```python
from build123d import *
from build123d.topology import SkipClean

# Parameters (mm, degrees)
SKETCH_1_R      = 1.9
SKETCH_1_R_2    = 2.7
SKETCH_1_R_3    = 2
EXTRUDE_1_DEPTH = 2.5
EXTRUDE_START   = -9
SKETCH_1_3_R    = 4.25
SKETCH_1_3_R_2  = 2.7
EXTRUDE_2_DEPTH = 9
SKETCH_2_R      = 3
SKETCH_2_R_2    = 1.9
EXTRUDE_4_DEPTH = 1
EXTRUDE_START_2 = 2.5
SKETCH_1_7_R    = 2.7
SKETCH_1_7_R_2  = 2
EXTRUDE_5_DEPTH = 10


with BuildPart() as part:
    # 草图1 → 凸台-拉伸1 (new body)
    with BuildSketch(Plane.XY):
        with BuildLine():
            ThreePointArc((-16.75, 33.05), (-19.75520382, 31.80520382), (-21, 28.8))
            Line((-21, 28.8), (-21, -28.8))
            ThreePointArc((-21, -28.8), (-19.75520382, -31.80520382), (-16.75, -33.05))
            Line((-16.75, -33.05), (16.75, -33.05))
            ThreePointArc((16.75, -33.05), (19.75520382, -31.80520382), (21, -28.8))
            Line((21, -28.8), (21, 28.8))
            ThreePointArc((21, 28.8), (19.75520382, 31.80520382), (16.75, 33.05))
            Line((16.75, 33.05), (-16.75, 33.05))
        make_face()
        with Locations((-12, 12)):
            Circle(SKETCH_1_R, mode=Mode.SUBTRACT)
        with Locations((-12, -12)):
            Circle(SKETCH_1_R, mode=Mode.SUBTRACT)
        with Locations((-16.75, 28.8)):
            Circle(SKETCH_1_R_2, mode=Mode.SUBTRACT)
        with Locations((-16.75, -28.8)):
            Circle(SKETCH_1_R_2, mode=Mode.SUBTRACT)
        with Locations((12, 12)):
            Circle(SKETCH_1_R, mode=Mode.SUBTRACT)
        with Locations((16.75, 28.8)):
            Circle(SKETCH_1_R_2, mode=Mode.SUBTRACT)
        with Locations((12, -12)):
            Circle(SKETCH_1_R, mode=Mode.SUBTRACT)
        with Locations((16.75, -28.8)):
            Circle(SKETCH_1_R_2, mode=Mode.SUBTRACT)
        Circle(SKETCH_1_R_3, mode=Mode.SUBTRACT)
    extrude(amount=EXTRUDE_1_DEPTH)

    # 草图1<3> → 凸台-拉伸2 (add)
    # profile 1 of 4: a face of its own
    with SkipClean():  # the faces are left unmerged after this step: merging them gives an invalid solid
        with BuildSketch(Plane.XY.offset(EXTRUDE_START)):
            with Locations(Location((-16.75, 28.8, 0), (0, 0, 180))):
                Circle(SKETCH_1_3_R)
            with Locations((-16.75, 28.8)):
                Circle(SKETCH_1_3_R_2, mode=Mode.SUBTRACT)
        # profile 2 of 4: a face of its own
        with BuildSketch(Plane.XY.offset(EXTRUDE_START)):
            with Locations(Location((-16.75, -28.8, 0), (0, 0, 180))):
                Circle(SKETCH_1_3_R)
            with Locations((-16.75, -28.8)):
                Circle(SKETCH_1_3_R_2, mode=Mode.SUBTRACT)
        # profile 3 of 4: a face of its own
        with BuildSketch(Plane.XY.offset(EXTRUDE_START)):
            with Locations((16.75, -28.8)):
                Circle(SKETCH_1_3_R)
            with Locations((16.75, -28.8)):
                Circle(SKETCH_1_3_R_2, mode=Mode.SUBTRACT)
        # profile 4 of 4: a face of its own
        with BuildSketch(Plane.XY.offset(EXTRUDE_START)):
            with Locations((16.75, 28.8)):
                Circle(SKETCH_1_3_R)
            with Locations((16.75, 28.8)):
                Circle(SKETCH_1_3_R_2, mode=Mode.SUBTRACT)
        extrude(amount=EXTRUDE_2_DEPTH)

    # 草图2 → 凸台-拉伸4 (add)
    # profile 1 of 4: a face of its own
    with SkipClean():  # the faces are left unmerged after this step: merging them gives an invalid solid
        with BuildSketch(Plane.XY.offset(2.5)):
            with Locations((-12, 12)):
                Circle(SKETCH_2_R)
            with Locations((-12, 12)):
                Circle(SKETCH_2_R_2, mode=Mode.SUBTRACT)
        # profile 2 of 4: a face of its own
        with BuildSketch(Plane.XY.offset(2.5)):
            with Locations(Location((12, 12, 0), (0, 0, 180))):
                Circle(SKETCH_2_R)
            with Locations(Location((12, 12, 0), (0, 0, 180))):
                Circle(SKETCH_2_R_2, mode=Mode.SUBTRACT)
        # profile 3 of 4: a face of its own
        with BuildSketch(Plane.XY.offset(2.5)):
            with Locations((12, -12)):
                Circle(SKETCH_2_R)
            with Locations((12, -12)):
                Circle(SKETCH_2_R_2, mode=Mode.SUBTRACT)
        # profile 4 of 4: a face of its own
        with BuildSketch(Plane.XY.offset(2.5)):
            with Locations(Location((-12, -12, 0), (0, 0, 180))):
                Circle(SKETCH_2_R)
            with Locations(Location((-12, -12, 0), (0, 0, 180))):
                Circle(SKETCH_2_R_2, mode=Mode.SUBTRACT)
        extrude(amount=EXTRUDE_4_DEPTH)

    # 草图1<7> → 凸台-拉伸5 (add)
    # profile 1 of 5: a face of its own
    with SkipClean():  # the faces are left unmerged after this step: merging them gives an invalid solid
        with BuildSketch(Plane.XY.offset(EXTRUDE_START_2)):
            with BuildLine():
                Line((-21, 8), (-18.046693311, 8))
                ThreePointArc((-18.046693311, 8), (-16.903570847, 17.34017724), (-7.5, 17.6844085))
                Line((-7.5, 17.6844085), (-7.5, 33.05))
                Line((-7.5, 33.05), (-16.75, 33.05))
                ThreePointArc((-16.75, 33.05), (-19.75520382, 31.80520382), (-21, 28.8))
                Line((-21, 28.8), (-21, 8))
            make_face()
            with Locations((-16.75, 28.8)):
                Circle(SKETCH_1_7_R, mode=Mode.SUBTRACT)
        # profile 2 of 5: a face of its own
        with BuildSketch(Plane.XY.offset(EXTRUDE_START_2)):
            with BuildLine():
                Line((-18.046693311, -8), (-21, -8))
                Line((-21, -8), (-21, -28.8))
                ThreePointArc((-21, -28.8), (-19.75520382, -31.80520382), (-16.75, -33.05))
                Line((-16.75, -33.05), (-7.5, -33.05))
                Line((-7.5, -33.05), (-7.5, -17.6844085))
                ThreePointArc((-7.5, -17.6844085), (-16.903570847, -17.34017724), (-18.046693311, -8))
            make_face()
            with Locations((-16.75, -28.8)):
                Circle(SKETCH_1_7_R, mode=Mode.SUBTRACT)
        # profile 3 of 5: a face of its own
        with BuildSketch(Plane.XY.offset(EXTRUDE_START_2)):
            with BuildLine():
                Line((7.5, 33.05), (7.5, 17.6844085))
                ThreePointArc((7.5, 17.6844085), (16.903570847, 17.34017724), (18.046693311, 8))
                Line((18.046693311, 8), (21, 8))
                Line((21, 8), (21, 28.8))
                ThreePointArc((21, 28.8), (19.75520382, 31.80520382), (16.75, 33.05))
                Line((16.75, 33.05), (7.5, 33.05))
            make_face()
            with Locations((16.75, 28.8)):
                Circle(SKETCH_1_7_R, mode=Mode.SUBTRACT)
        # profile 4 of 5: a face of its own
        with BuildSketch(Plane.XY.offset(EXTRUDE_START_2)):
            with BuildLine():
                Line((7.5, -17.6844085), (7.5, -33.05))
                Line((7.5, -33.05), (16.75, -33.05))
                ThreePointArc((16.75, -33.05), (19.75520382, -31.80520382), (21, -28.8))
                Line((21, -28.8), (21, -8))
                Line((21, -8), (18.046693311, -8))
                ThreePointArc((18.046693311, -8), (16.903570847, -17.34017724), (7.5, -17.6844085))
            make_face()
            with Locations((16.75, -28.8)):
                Circle(SKETCH_1_7_R, mode=Mode.SUBTRACT)
        # profile 5 of 5: a face of its own
        with BuildSketch(Plane.XY.offset(EXTRUDE_START_2)):
            with BuildLine():
                ThreePointArc((12.000001775, 0), (3.514719253, 3.514717998), (0, 12))
                ThreePointArc((0, 12), (-3.514717998, 3.514717478), (-12, -1.775e-06))
                ThreePointArc((-12, -1.775e-06), (-3.514717478, -3.514719773), (1.775e-06, -12.000001775))
                ThreePointArc((1.775e-06, -12.000001775), (3.514719773, -3.514719253), (12.000001775, 0))
            make_face()
            Circle(SKETCH_1_7_R_2, mode=Mode.SUBTRACT)
        extrude(amount=EXTRUDE_5_DEPTH)


solid = part.part
```
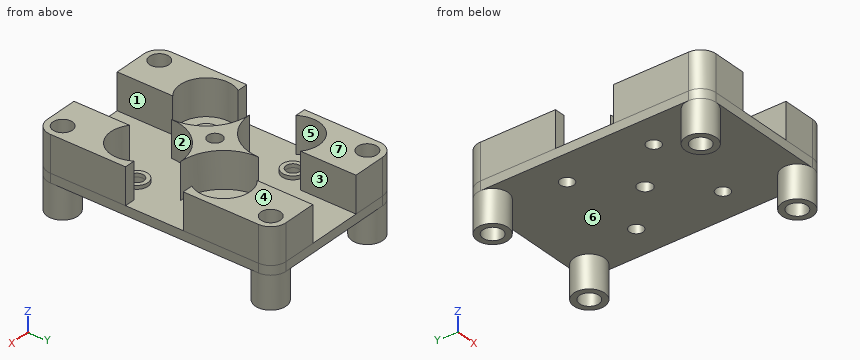
Work out the finished part from the listing and answer in its coordinate system (mm). Face numbers are marked on the shaded views. A direction names the side the tool comes from. Give positions to 0.01 mm unless a question says otherwise; leave off trailing zeros. Order: outer loops, then holes, each group sorted by start corner. A loop starts at its lowest first (then second) coordinate and runs counter-clockwise, first axis right, second up. Notation, with made-up numbers: M -13.5,75 L 22.5,75 A7 ccw 22.5,82 Z; hole C -36.5,84.5 d2. An arc over 180 degrees is marked long. Return JSON: item names as keys, results as strings.
1) A tool of negligible diameter and unlimited length cuts with its end or side. For the marked faces 1, 2, 3 and 4, from which of +Z, -Z, +X, -X, +Y, -Y can it reach the whole face along a straight path? Write none if from no direction.
Resolved:
{"face 1": "+Z, -Y", "face 2": "+Z", "face 3": "+Z, +Y", "face 4": "+Z, +X, -X, +Y, -Y"}
2) Each of these flat-tipped pins is pushed along its axis until it touches: pin 1 (6 mm diameter, centred on x = 12, y = -12, fed in from -Z); pin 2 (4 mm diameter, centred on x = -4, z = 8.5, fed in from +Y); pin 3 (3 mm diameter, centred on x = 11, y = 11.5, fed in from +Z). Where does it stop, or does it pass through?
Resolved:
{"pin 1": "z = 0", "pin 2": "y = 5.37", "pin 3": "z = 3.5"}
3) Section B-B, the plane z = -4.5 is taken. Write down the section's boundary in (x, y), plus the area to 3 significant figures.
Resolved:
{"outline": "C -16.75,-28.8 d8.5; C -16.75,28.8 d8.5; C 16.75,-28.8 d8.5; C 16.75,28.8 d8.5; hole C -16.75,-28.8 d5.4; hole C -16.75,28.8 d5.4; hole C 16.75,-28.8 d5.4; hole C 16.75,28.8 d5.4", "area": "135 mm^2"}
4) For a pull along X with two mould halves and no side action, classify the marked faces 5, 6 and 7 as +X half, -X half, draft (parallel to the pull), parting line (faces both ways), or undercut.
Resolved:
{"face 5": "undercut", "face 6": "undercut", "face 7": "draft"}
5) Section C-C, the plane y = -20 is taken. Write down the section's boundary in (x, z), plus the area to 3 significant figures.
Resolved:
{"outline": "M -21,0 L 21,0 L 21,12.5 L 7.5,12.5 L 7.5,2.5 L -7.5,2.5 L -7.5,12.5 L -21,12.5 Z", "area": "375 mm^2"}
6) Section A-A, the plane z = 4.5 is taken. Give the number of separate pieces and of enclosed holes in the cut face, plus the area to 3 significant figures.
Resolved:
{"separate pieces": "5", "enclosed holes": "5", "area": "888 mm^2"}
7) Section D-D, the plane y = 11 is taken. Write down the section's boundary in (x, z).
Resolved:
{"outline": "M -21,0 L -13.62,0 L -13.62,3.5 L -14.83,3.5 L -14.83,2.5 L -19.18,2.5 L -19.18,12.5 L -21,12.5 Z; M -10.38,0 L 10.38,0 L 10.38,3.5 L 9.17,3.5 L 9.17,2.5 L 0.04,2.5 L 0.04,12.5 L -0.04,12.5 L -0.04,2.5 L -9.17,2.5 L -9.17,3.5 L -10.38,3.5 Z; M 13.62,0 L 21,0 L 21,12.5 L 19.18,12.5 L 19.18,2.5 L 14.83,2.5 L 14.83,3.5 L 13.62,3.5 Z"}
8) Straight lines are drawn through the part: line 1 along X through (y, z) = (20, 5.75); line 2 along Y through (x, z) = (12, 1.85); line 3 along X through (y, z) = (29.5, 8). For each, find the intervals that lie inside material, in ascending order. Write a range as [from, to].
Resolved:
{"line 1": "[-21, -7.5], [7.5, 21]", "line 2": "[-33.05, -13.9], [-10.1, 10.1], [13.9, 33.05]", "line 3": "[-20.94, -19.36], [-14.14, -7.5], [7.5, 14.14], [19.36, 20.94]"}
